The figure shows three views and two pictorial views of one solid part (mm, origin at its lowest corner). Answer the questions. Round coordinates to 2 decimals unless told otherwise and drop trailing zeros. Loops run counter-clockwise (first coordinate to the right, second up) from the corner with the lowest first, then second, coordinate; pieces in that order, holes last. Notation, with made-up numbers: (54.25, -3) -> (103.25, -3) arc R14 cw to (103.25, 5) -> close; hole circle Ø2 at (47, 28.25). An arc over 180 degrees is marked (long way). Use a Markdown table: item, result. Add a question column.
Q1. Section A-A on x = 15 is taken. Give the vertices of the cut face in (y, z), then the cut area to 3 significant figures.
Q2. Consider line 1 (Y direction, x = 15, z = 1.1); line 2 (X direction, y = 43.5, z = 1.1); line 3 (Y direction, x = 18, z = 0.95). Determine where each line is inside the solid, lowest interval first.
Q3. Given pin 1 Ø12 at (x, y) = (36, 17) entering from -Z; pin 2 Ø6 at (x, y) = (45, 15) entering from +Z, each flat-ended and moving along its own axis, determine where each tip first touches the part or whether it passes through.
Q4. Section C-C on z = 1.2 is taken. Give the vertices of the cut face in (x, y).
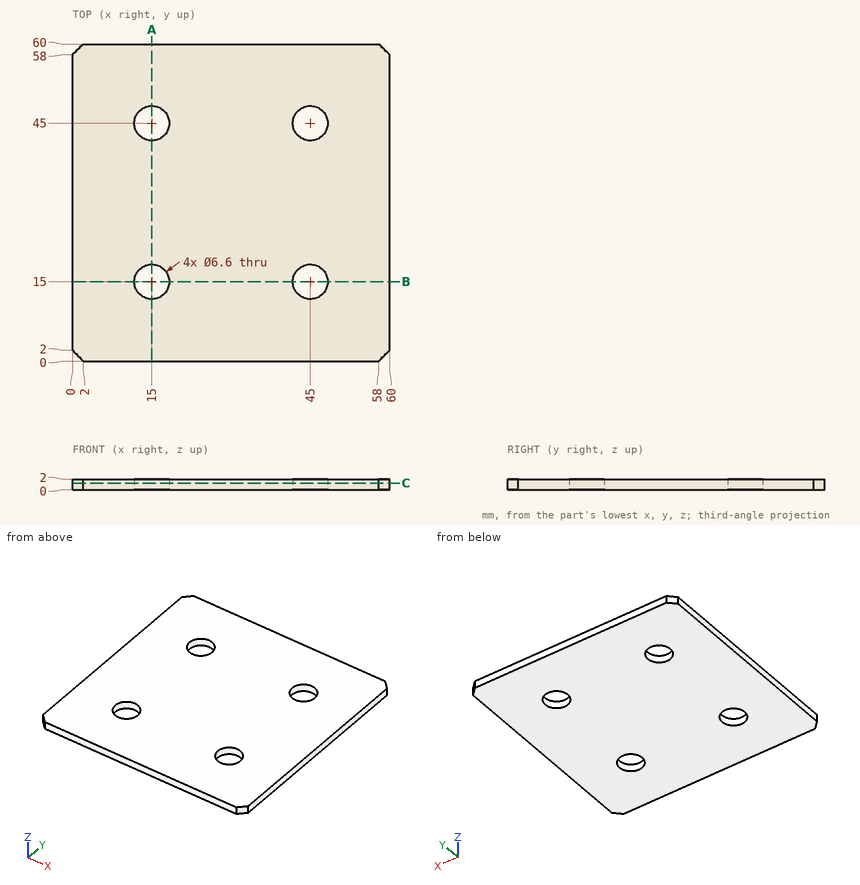
Checked values:
| question | item | result |
|---|---|---|
| 1 | outline | (0, 0) -> (11.7, 0) -> (11.7, 2) -> (0, 2) -> close; (18.3, 0) -> (41.7, 0) -> (41.7, 2) -> (18.3, 2) -> close; (48.3, 0) -> (60, 0) -> (60, 2) -> (48.3, 2) -> close |
| 1 | area | 93.6 mm2 |
| 2 | line 1 | y = 0 to 11.7, 18.3 to 41.7, 48.3 to 60 |
| 2 | line 2 | x = 0 to 12.06, 17.94 to 42.06, 47.94 to 60 |
| 2 | line 3 | y = 0 to 13.63, 16.37 to 43.63, 46.37 to 60 |
| 3 | pin 1 | stops at z = 0 |
| 3 | pin 2 | passes through |
| 4 | outline | (0, 2) -> (2, 0) -> (58, 0) -> (60, 2) -> (60, 58) -> (58, 60) -> (2, 60) -> (0, 58) -> close; hole circle Ø6.6 at (15, 15); hole circle Ø6.6 at (15, 45); hole circle Ø6.6 at (45, 15); hole circle Ø6.6 at (45, 45) |
